Print and shaded views of the part. All mm, measured from the part's lowest x, y and z. Coordinates: 2 decimals unless noted, no trailing zeros. Loops run counter-clockwise (first coordinate to the right, second up) from the corner with the lowest first, then second, coordinate; pieces in that order, holes last.
1) Saw through at B-B, the plane x = 6.35. Write the cut outline in (y, z).
2) Two-plate mould, pull along Y, no slides. Class the marked faces 1, 2 and 3: +Y half, -Y half, draft (parallel to the pull), parting line (faces both ways), or undercut.
3) Wall check: line 1 along Y through (x, z) = (6.5, 1.3) (1 decimal); line 2 along Y through (x, z) = (5.25, 0.4); line 3 along X through (y, z) = (20.5, 0.8) (1 decimal). Give the ranges that are in metal, low to high.
4) Saw through at C-C, the plane y = 6.35. Write the cut outline in (x, z), and give its area (3 significant figures).
5) Saw through at D-D, the plane x = 8. Write the cut outline in (y, z).
6) Saw through at A-A, the plane z = 0.55. Give the number of separate pieces and of enclosed holes in the cut face, and give its area (3 significant figures).
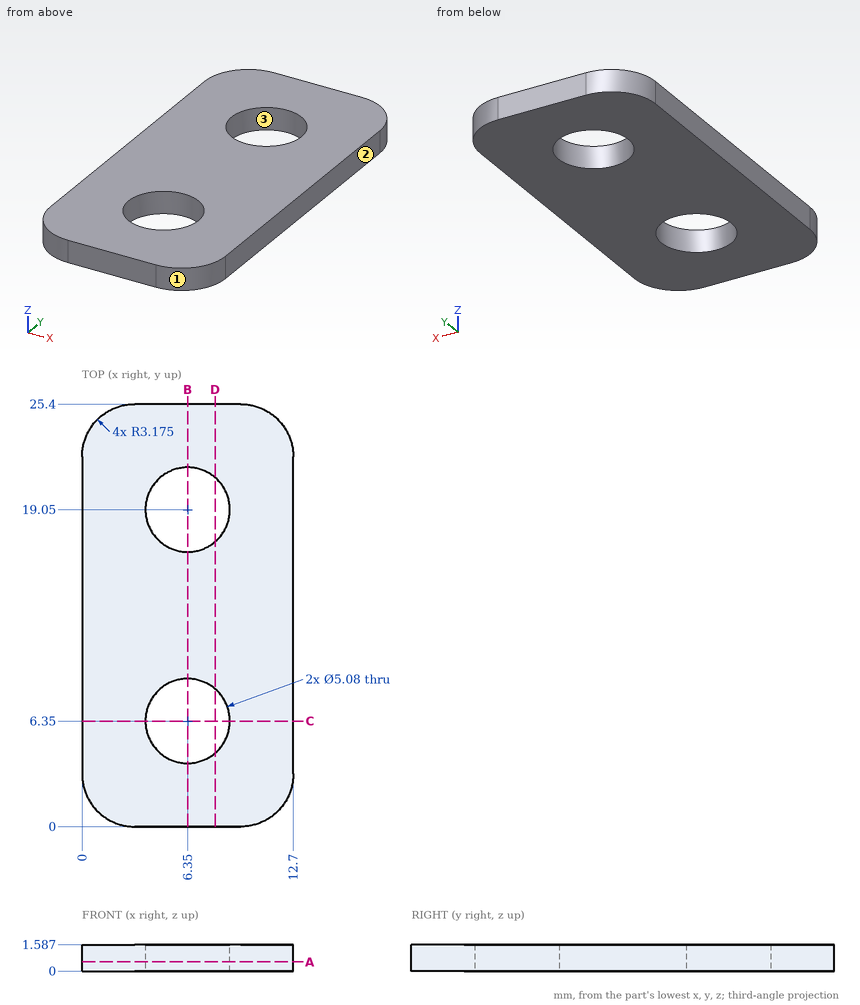
Data:
1. outline: (0, 0) - (3.81, 0) - (3.81, 1.59) - (0, 1.59) - close; (8.89, 0) - (16.51, 0) - (16.51, 1.59) - (8.89, 1.59) - close; (21.59, 0) - (25.4, 0) - (25.4, 1.59) - (21.59, 1.59) - close
2. face 1: -Y half
2. face 2: draft
2. face 3: undercut
3. line 1: y = 0 to 3.8, 8.9 to 16.5, 21.6 to 25.4
3. line 2: y = 0 to 4.06, 8.64 to 16.76, 21.34 to 25.4
3. line 3: x = 0 to 4.3, 8.4 to 12.7
4. outline: (0, 0) - (3.81, 0) - (3.81, 1.59) - (0, 1.59) - close; (8.89, 0) - (12.7, 0) - (12.7, 1.59) - (8.89, 1.59) - close
4. area: 12.1 mm2
5. outline: (0, 0) - (4.42, 0) - (4.42, 1.59) - (0, 1.59) - close; (8.28, 0) - (17.12, 0) - (17.12, 1.59) - (8.28, 1.59) - close; (20.98, 0) - (25.4, 0) - (25.4, 1.59) - (20.98, 1.59) - close
6. separate pieces: 1
6. enclosed holes: 2
6. area: 273 mm2
